Input: dimensioned drawing with shaded views. Units: mm. Origin: part minimum x, y, z. Give positions to 0.01 mm unless a question says otherwise; leave off trailing zeros. Order: outer loops, then holes, each group sorted by start corner. A loop starts at its lowest first (then second) coordinate and runs counter-clockwise, first axis right, second up.
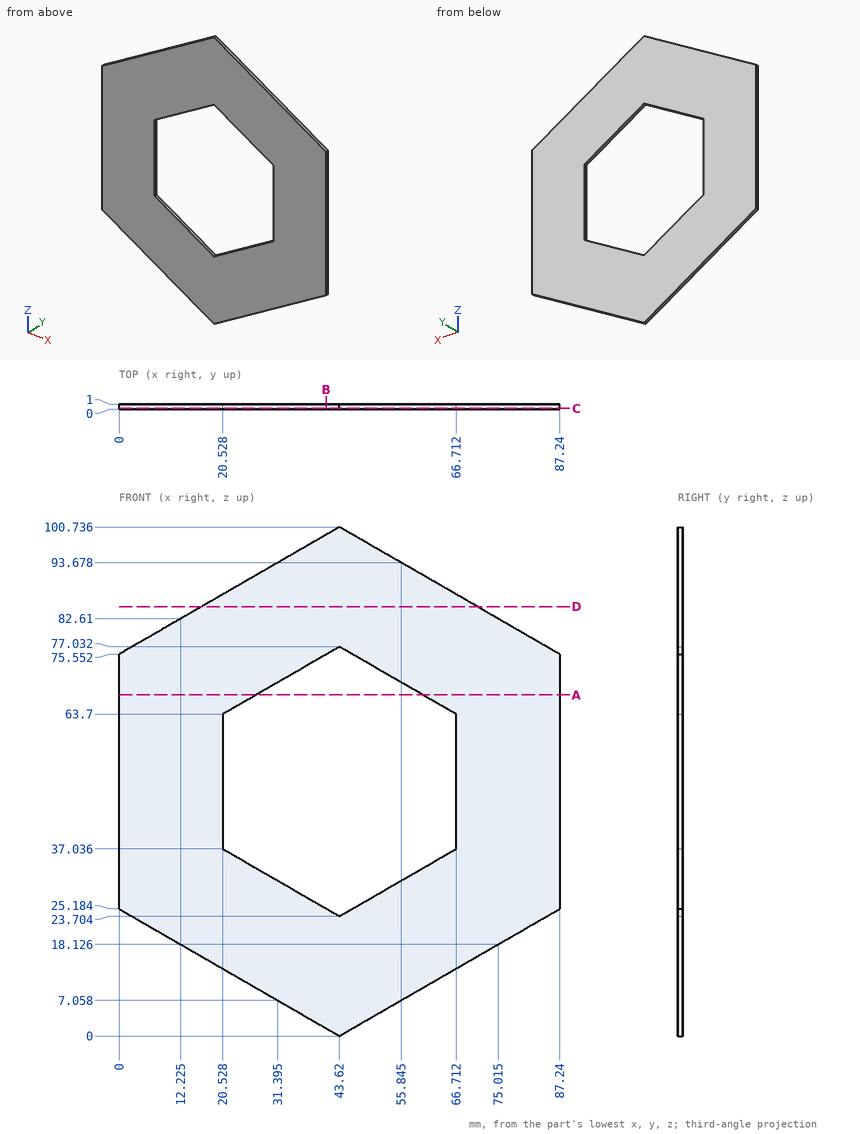
1) Section query A-A, the plane z = 67.5. Return the cut outline in (x, y).
Report:
outline: (0, 0) - (27.11, 0) - (27.11, 1) - (0, 1) - close; (60.13, 0) - (87.24, 0) - (87.24, 1) - (60.13, 1) - close
2) Section query B-B, the plane x = 41. Return the cut outline in (y, z).
Report:
outline: (0, 1.51) - (1, 1.51) - (1, 25.22) - (0, 25.22) - close; (0, 75.52) - (1, 75.52) - (1, 99.22) - (0, 99.22) - close
3) Section query D-D, the plane z = 85. Return the cut outline in (x, y) (1 decimal).
Report:
outline: (16.4, 0) - (70.9, 0) - (70.9, 1) - (16.4, 1) - close
4) Material intervals for L1, parallel to X at y = 0.4, z = 42.5; L2, parallel to Z at x = 49, y = 0.3 (1 decimal); L3, parallel to X at y = 0.95, z = 69, sorted ascending.
Report:
L1: x = 0 to 20.53, 66.71 to 87.24
L2: z = 3.1 to 26.8, 73.9 to 97.6
L3: x = 0 to 29.71, 57.53 to 87.24
5) Section query C-C, the plane y = 0.15. Return the cut outline in (x, z) (1 decimal).
Report:
outline: (0, 25.2) - (43.6, 0) - (87.2, 25.2) - (87.2, 75.6) - (43.6, 100.7) - (0, 75.6) - close; hole (20.5, 37) - (43.6, 23.7) - (66.7, 37) - (66.7, 63.7) - (43.6, 77) - (20.5, 63.7) - close
